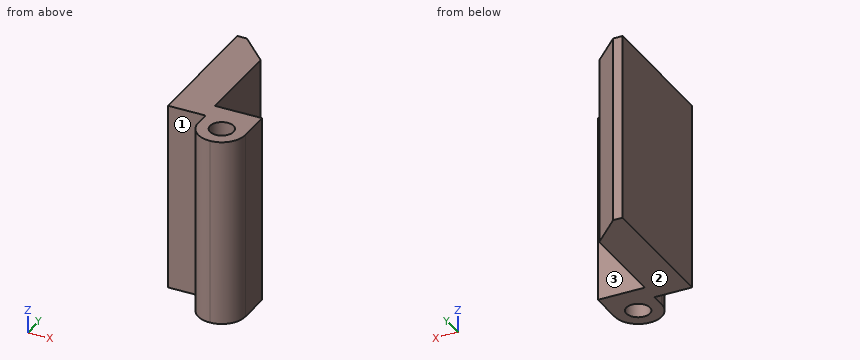
Autodesk Inventor part; units mm, degrees
ref_plane "YZ Plane" through (0, 0, 0) normal (1, 0, 0) x (0, 1, 0)
ref_plane "XZ Plane" through (0, 0, 0) normal (0, 1, 0) x (-1, 0, 0)
ref_plane "XY Plane" through (0, 0, 0) normal (0, 0, 1) x (1, 0, 0)
sketch "Sketch1" plane through (0, 0, 0) normal (0, 0, 1) x (1, 0, 0)
  line L0 (0, 0) -> (18, 0)
  line L1 (18, 0) -> (18, 32)
  line L2 (18, 32) -> (0, 32)
  line L3 (0, 32) -> (0, 0)
  dimension "d0" = 18
  dimension "d1" = 32
extrude "Extrusion1" add sketch "Sketch1" along normal blind 40
sketch "Sketch2" plane through (0, 0, 40) normal (0, 0, 1) x (1, 0, 0)
  point P0 (0, 0)
sketch "Sketch3" plane through (0, 32, 0) normal (0, 1, 0) x (1, 0, 0)
  line L0 (18, -40) -> (8, -40)
  line L1 (8, -40) -> (8, 0)
  line L2 (8, 0) -> (18, 0)
  line L3 (18, 0) -> (18, -40)
  point P0 (0, 0)
  dimension "d4" = 10
  dimension "d5" = 40
extrude "Extrusion2" cut sketch "Sketch3" against normal blind 20
sketch "Sketch4" plane through (0, 0, 40) normal (0, 0, 1) x (1, 0, 0)
  line L0 (0, 32) -> (0, 0)
  line L1 (0, 0) -> (8, 0)
  line L2 (8, 0) -> (8, 8)
  line L3 (8, 8) -> (0, 8)
  line L4 (0, 8) -> (0, 0)
  dimension "d8" = 8
  dimension "d9" = 8
extrude "Extrusion3" cut sketch "Sketch4" against normal blind 40
fillet "Fillet1" radius 5 2 edges at (18, 0, 20) (8, 0, 20)
sketch "Sketch5" plane through (0, 0, 40) normal (0, 0, 1) x (1, 0, 0)
  arc A0 (8, 5) -> (18, 5) centre (13, 5) ccw
  circle A1 centre (13, 5) radius 2.5
  point P0 (0, 0)
  dimension "d13" = 5
extrude "Extrusion4" cut sketch "Sketch5" against normal blind 40
sketch "Sketch6" plane through (0, 32, 40) normal (0, 1, 0) x (1, 0, 0)
  line L0 (0, 0) -> (8, 0)
  line L1 (8, 0) -> (8, 40)
  line L2 (0, 0) -> (8, 0)
  line L3 (8, 0) -> (8, 40)
  line L4 (8, 40) -> (0, 40)
  line L5 (0, 40) -> (0, 0)
extrude "Extrusion5" add sketch "Sketch6" along normal blind 5
sketch "Sketch7" plane through (0, 0, 40) normal (0, 0, 1) x (1, 0, 0)
  line L0 (8, 37) -> (0, 37)
  line L1 (2, 37) -> (8, 31)
  line L2 (8, 37) -> (8, 12)
  point P0 (0, 0)
  dimension "d18" = 6
extrude "Extrusion6" cut sketch "Sketch7" against normal blind 40
properties part number "Hinge"
Geometry check sheet. Reference: the model listing, model coordinates, mm. Face numbers are marked on the shaded views. A direction names the side the tool comes from. Round coordinates to 2 decimals unless told otherwise and drop trailing zeros. Write each loop counter-clockwise with the first axis right and the second up, starting at its lowest first coordinate (ties: lowest second). Pieces come first, ordered by that corner, then holes. Notation, with made-up numbers: (-38, -19.5) - (20, -19.5) arc R20 cw to (20, -10.5) - close; hole circle Ø5 at (63, 46.5). An arc over 180 degrees is marked (long way). One line per item, written item: value.
1. Scan lines: L1, parallel to Y at x = 13, z = 12; L2, parallel to X at y = 26, z = 2.5; L3, parallel to Y at x = 12.5, z = 24. Record each from-to range of solid material in increasing order.
The answers:
L1: y = 0 to 2.5, 7.5 to 12
L2: x = 0 to 8
L3: y = 0.03 to 2.55, 7.45 to 12
2. Cross-section at D-D on y = 24.5. Record the boundary of the cut face in (x, z).
The answers:
outline: (0, 0) - (8, 0) - (8, 40) - (0, 40) - close
3. Cross-section at A-A on y = 4. Record the boundary of the cut face in (x, z), and give its area (3 significant figures).
The answers:
outline: (8.1, 0) - (10.71, 0) - (10.71, 40) - (8.1, 40) - close; (15.29, 0) - (17.9, 0) - (17.9, 40) - (15.29, 40) - close
area: 209 mm^2
4. Set-up check for the marked faces 1, 2 and 3: record each of +Z, -Z, +X, -X, +Y, -Y from which the full face is reachable in a straight line by a thin tool's end or side.
The answers:
face 1: +Z, -Z, -X, -Y
face 2: -Z, +X, -X, +Y, -Y
face 3: +Z, -Z, +X, +Y
5. Depth check by flat-ended pin: pin 1 Ø2.5 at (x, z) = (2, 15.5) entering from -Y; pin 2 Ø3 at (x, z) = (12, 12) entering from +Y; pin 3 Ø8 at (x, z) = (7.5, 25) entering from +Y. Enter the tip coordinate at first touch or a pass-through.
The answers:
pin 1: stops at y = 8
pin 2: stops at y = 12
pin 3: stops at y = 35.5
6. Cross-section at C-C on x = 5.5. Record the boundary of the cut face in (y, z), and give its area (3 significant figures).
The answers:
outline: (8, 0) - (33.5, 0) - (33.5, 40) - (8, 40) - close
area: 1,020 mm^2
